The model under review builds one solid part; all positions refer to its coordinate system, in mm. A direction names the side the tool comes from. Coordinates: 2 decimals unless noted, no trailing zeros. Write each loop counter-clockwise with the first axis right and the second up, starting at its lowest first coordinate (ties: lowest second). Pieces come first, ordered by that corner, then holes. Notation, with made-up numbers: (70, 54.25) - (118, 54.25) arc R29 cw to (118, 93.25) - close; hole circle Ø9 at (-36.5, 11.25). An arc over 180 degrees is marked (long way). Put each result on its own line as item: value.
from build123d import *

# Parameters (mm, degrees)
BASE_FLANGE1_DEPTH = 871.6
CUT_EXTRUDE1_DEPTH = 10


# Sheet-metal steps are written as plain solids
with BuildPart() as part:
    # Sketch1 → Base-Flange1 (new body)
    with BuildSketch(Plane(origin=(0, 0, 0), x_dir=(1, 0, 0), z_dir=(0, 1, 0))):
        with BuildLine():
            Line((-231, 460), (-231, 383.6))
            ThreePointArc((-231, 383.6), (-230.53137085, 382.46862915), (-229.4, 382))
            Line((-229.4, 382), (311, 382))
            ThreePointArc((311, 382), (337.870057685, 370.870057685), (349, 344))
            Line((349, 344), (349, -600))
            ThreePointArc((349, -600), (337.870057685, -626.870057685), (311, -638))
            Line((311, -638), (269, -638))
            Line((269, -638), (269, -638.8))
            Line((269, -638.8), (311, -638.8))
            ThreePointArc((311, -638.8), (338.43574311, -627.43574311), (349.8, -600))
            Line((349.8, -600), (349.8, 344))
            ThreePointArc((349.8, 344), (338.43574311, 371.43574311), (311, 382.8))
            Line((311, 382.8), (-229.4, 382.8))
            ThreePointArc((-229.4, 382.8), (-229.965685425, 383.034314575), (-230.2, 383.6))
            Line((-230.2, 383.6), (-230.2, 460))
            Line((-230.2, 460), (-231, 460))
        make_face()
    extrude(amount=BASE_FLANGE1_DEPTH)

    # Sketch4 → Cut-Extrude1 (cut)
    with BuildSketch(Plane(origin=(-230.2, 0, 0), x_dir=(0, 0, -1), z_dir=(1, 0, 0))):
        with BuildLine():
            Line((460, 871.6), (385, 871.6))
            ThreePointArc((385, 871.6), (438.033008589, 849.633008589), (460, 796.6))
            Line((460, 796.6), (460, 871.6))
        make_face()
        with BuildLine():
            Line((460, 0), (385, 0))
            ThreePointArc((385, 0), (438.033008589, 21.966991411), (460, 75))
            Line((460, 75), (460, 0))
        make_face()
    extrude(amount=-CUT_EXTRUDE1_DEPTH, mode=Mode.SUBTRACT)


solid = part.part
1. For pin 1 Ø1 at (x, y) = (62, 773) entering from -Z; pin 2 Ø8 at (y, z) = (224, -296) entering from -X; pin 3 Ø8 at (x, y) = (124.5, 487.5) entering from +Z, all flat-tipped, find the tip position at first contact; note any pin that passes through.
Determined:
pin 1: stops at z = -382.8
pin 2: stops at x = 349
pin 3: stops at z = -382
2. The part is to be moulded in two halves that separate along Z. For faces 4 (the flat face through (-230.2, 430, -421)), 5 (the cylindrical face through (338.164, 429.699, 626.573)), 6 (the cylindrical face through (337.573, 429.699, -371.164)), 7 (the cylindrical face through (338.74, 429.7, -371.13)), say which applies: +Z half, -Z half, draft (parallel to the pull), parting line (faces both ways), or undercut.
Determined:
face 4: draft
face 5: undercut
face 6: undercut
face 7: -Z half
3. Consider section A-A on y = 300.5. State the section outline as (x, z) points.
Determined:
outline: (-231, -460) - (-230.2, -460) - (-230.2, -383.6) arc R0.8 cw to (-229.4, -382.8) - (311, -382.8) arc R38.8 ccw to (349.8, -344) - (349.8, 600) arc R38.8 ccw to (311, 638.8) - (269, 638.8) - (269, 638) - (311, 638) arc R38 cw to (349, 600) - (349, -344) arc R38 cw to (311, -382) - (-229.4, -382) arc R1.6 ccw to (-231, -383.6) - close
4. To check wall thickness, follow probe 1 along Z at (x, y) = (209, 347); probe 2 along X at (y, z) = (655.5, -263). State the ranges of each line that lie inside material, in increasing order.
Determined:
probe 1: z = -382.8 to -382
probe 2: x = 349 to 349.8
5. Machinability: for faces 1 (the flat face through (45, 430, -382.8)), 2 (the flat face through (290, 430, 638)), 3 (the flat face through (-231, 430, -422)), which of the approach directions +Z, -Z, +X, -X, +Y, -Y give a long, thin tool a straight path to every point of the face, cutting with its end or side? Answer none if there is none.
Determined:
face 1: -Z, +X, +Y, -Y
face 2: -X, +Y, -Y
face 3: +Z, -Z, -X, +Y, -Y
6. Consider section C-C on x = 198.5. State the section outline as (y, z) points.
Determined:
outline: (0, -382.8) - (871.6, -382.8) - (871.6, -382) - (0, -382) - close
7. Consider section B-B on z = 295. State the section outline as (x, y) points, plus the area to 3 significant figures.
Determined:
outline: (349, 0) - (349.8, 0) - (349.8, 871.6) - (349, 871.6) - close
area: 697 mm^2
